from build123d import *

# Parameters (mm, degrees)
SKETCH2_R               = 6
BOSS_EXTRUDE1_DEPTH     = 4
SKETCH3_W               = 5
SKETCH3_H               = 30
BOSS_EXTRUDE3_DEPTH     = 24
BOSS_EXTRUDE5_DEPTH     = 5
SKETCH7_3_R             = 3.25755
CUT_EXTRUDE3_DEPTH      = 5
FILLET3_R               = 10
CUT_EXTRUDE4_DEPTH      = 25
CUT_EXTRUDE4_DEPTH_BACK = 1
SKETCH8_R               = 7.5
CUT_EXTRUDE5_DEPTH      = 50.515905416
CUT_EXTRUDE5_DEPTH_BACK = 50.515905416
SKETCH9_R               = 2.75
FILLET4_R               = 1
BOSS_EXTRUDE6_DEPTH     = 4
FILLET6_R               = 2
BOSS_EXTRUDE7_DEPTH     = 4


with BuildPart() as part:
    # Sketch2 → Boss-Extrude1 (new body)
    with BuildSketch(Plane(origin=(0, 0, 0), x_dir=(1, 0, 0), z_dir=(0, 1, 0))):
        with BuildLine():
            Line((18.000912404, -14.946929254), (18.000912404, 15.053070746))
            Line((18.000912404, 15.053070746), (0.039090451, 15.053070746))
            ThreePointArc((0.039090451, 15.053070746), (-10.199781301, 11.024824414), (-14.94907539, 1.099832277))
            ThreePointArc((-14.94907539, 1.099832277), (-10.959209921, -10.21234771), (0.039090451, -15.000022662))
            Line((0.039090451, -15.000022662), (10.151696986, -14.946929254))
            Line((10.151696986, -14.946929254), (18.000912404, -14.946929254))
        make_face()
        with Locations(Location((0.000957071, 0.012970337, 0), (0, 0, 270))):
            Circle(SKETCH2_R, mode=Mode.SUBTRACT)
    boss_extrude1 = extrude(amount=BOSS_EXTRUDE1_DEPTH)

    # Sketch3 → Boss-Extrude3 (add)
    with BuildSketch(Plane(origin=(0, 4, 0), x_dir=(1, 0, 0), z_dir=(0, 1, 0))):
        with Locations((15.500912404, 0.053070746)):
            Rectangle(SKETCH3_W, SKETCH3_H)
    extrude(amount=BOSS_EXTRUDE3_DEPTH)

    # Mirror1: Boss-Extrude1 across plane
    add(boss_extrude1.mirror(Plane.ZX.offset(16)))

    # Sketch7 → Boss-Extrude5 (add)
    with BuildSketch(Plane.ZY.offset(-13.000912404)):
        with BuildLine():
            Line((-15.053070746, 0), (-15.053070746, 4))
            Line((-15.053070746, 4), (-15.053070746, 7.075913265))
            ThreePointArc((-15.053070746, 7.075913265), (-18.310620746, 10.333463265), (-15.053070746, 13.591013265))
            Line((-15.053070746, 13.591013265), (-15.053070746, 20.666926531))
            ThreePointArc((-15.053070746, 20.666926531), (-25.386534011, 10.333463265), (-15.053070746, 0))
        make_face()
        with BuildLine():
            ThreePointArc((25.146929254, 21.8), (22.159418422, 29.012489168), (14.946929254, 32))
            Line((14.946929254, 32), (14.946929254, 28))
            Line((14.946929254, 28), (14.946929254, 25.05755))
            ThreePointArc((14.946929254, 25.05755), (17.250364949, 24.103435695), (18.204479254, 21.8))
            ThreePointArc((18.204479254, 21.8), (17.250364949, 19.496564305), (14.946929254, 18.54245))
            Line((14.946929254, 18.54245), (14.946929254, 11.6))
            ThreePointArc((14.946929254, 11.6), (22.159418422, 14.587510832), (25.146929254, 21.8))
        make_face()
        with BuildLine():
            Line((14.946929254, 28), (14.946929254, 32))
            ThreePointArc((14.946929254, 32), (4.746929254, 21.8), (14.946929254, 11.6))
            Line((14.946929254, 11.6), (14.946929254, 18.54245))
            ThreePointArc((14.946929254, 18.54245), (11.689379254, 21.8), (14.946929254, 25.05755))
            Line((14.946929254, 25.05755), (14.946929254, 28))
        make_face()
    extrude(amount=-BOSS_EXTRUDE5_DEPTH)

    # Sketch7<3> → Cut-Extrude3 (cut)
    with BuildSketch(Plane.ZY.offset(-13.000912404)):
        with Locations((14.946929254, 21.8)):
            Circle(SKETCH7_3_R)
        with Locations((-15.053070746, 10.333463265)):
            Circle(SKETCH7_3_R)
    extrude(amount=-CUT_EXTRUDE3_DEPTH, mode=Mode.SUBTRACT)

    # Fillet3
    # the kernel refuses this fillet: 10 mm, written as the material it adds along each edge
    with BuildSketch(Plane(origin=(13.000912404, 20.666926531, -15.053070746), x_dir=(0, -0.25425566101904284, -0.9671370424297528), z_dir=(1, 0, 0))) as fillet3_piece_1:
        with BuildLine():
            CenterArc((7.797239676, 9.671370424), FILLET3_R, 194.729484057, 60.541031886)
            Line((-1.874130748, 7.128813814), (0, 0))
            ThreePointArc((0, 0), (2.627341533, 0.339588165), (5.254683066, 0))
        make_face()
    extrude(amount=5)
    with BuildSketch(Plane(origin=(13.000912404, 11.6, 14.946929254), x_dir=(0, -1, 0), z_dir=(1, 0, 0))) as fillet3_piece_2:
        with BuildLine():
            CenterArc((7.351068344, -10), FILLET3_R, 90, 60.326985198)
            ThreePointArc((-1.337579351, -5.04950495), (-0.340063626, -2.611829759), (0, 0))
            Line((0, 0), (7.351068344, 0))
        make_face()
    extrude(amount=5)

    # Sketch8 → Cut-Extrude4 (cut, two sides: drawn at the far end of the back side and taken through both)
    with BuildSketch(Plane(origin=(0, 4, 0), x_dir=(1, 0, 0), z_dir=(0, 1, 0)).offset(-CUT_EXTRUDE4_DEPTH_BACK)):
        with Locations(Location((0, 0, 0), (0, 0, 90))):
            Circle(SKETCH8_R)
    extrude(amount=CUT_EXTRUDE4_DEPTH + CUT_EXTRUDE4_DEPTH_BACK, mode=Mode.SUBTRACT)

    # Sketch9 → Cut-Extrude5 (cut, two sides: drawn at the far end of the back side and taken through both)
    with BuildSketch(Plane.ZY.offset(-13.000912404).offset(-CUT_EXTRUDE5_DEPTH_BACK)):
        with Locations((9, 10.2)):
            Circle(SKETCH9_R)
        with Locations((-9, 21.8)):
            Circle(SKETCH9_R)
    extrude(amount=CUT_EXTRUDE5_DEPTH + CUT_EXTRUDE5_DEPTH_BACK, mode=Mode.SUBTRACT)

    # Fillet4
    fillet4_edges = [part.edges().sort_by_distance(p)[0] for p in [
        (13.000912404, 4, -0.053070746),
        (13.000912404, 28, -0.053070746),
    ]]
    fillet(fillet4_edges, radius=FILLET4_R)

    # Sketch10 → Boss-Extrude6 (add)
    with BuildSketch(Plane.XZ):
        with BuildLine():
            ThreePointArc((0.039090451, -15.053070746), (-5.733491903, -13.900038334), (-10.620178824, -10.617892431))
            Line((-10.620178824, -10.617892431), (-9.005905934, -15.053070746))
            Line((-9.005905934, -15.053070746), (0.039090451, -15.053070746))
        make_face()
        with BuildLine():
            ThreePointArc((-10.571777141, 10.613334735), (-5.701848976, 13.860114152), (0.039090451, 15.000022662))
            Line((0.039090451, 15.000022662), (-8.957960629, 15.047259158))
            Line((-8.957960629, 15.047259158), (-10.571777141, 10.613334735))
        make_face()
    extrude(amount=-BOSS_EXTRUDE6_DEPTH)

    # Fillet6
    fillet6_edges = [part.edges().sort_by_distance(p)[0] for p in [
        (-9.005905934, 2, -15.053070746),
        (-8.957960629, 2, 15.047259158),
    ]]
    fillet(fillet6_edges, radius=FILLET6_R)

    # Sketch11 → Boss-Extrude7 (add)
    with BuildSketch(Plane(origin=(0, 32, 0), x_dir=(1, 0, 0), z_dir=(0, 1, 0))):
        with BuildLine():
            ThreePointArc((0.039090451, -15.000022662), (-5.701848976, -13.860114152), (-10.571777141, -10.613334735))
            Line((-10.571777141, -10.613334735), (-9.439611791, -13.723933469))
            ThreePointArc((-9.439611791, -13.723933469), (-8.703074785, -14.681202997), (-7.549726254, -15.039865618))
            Line((-7.549726254, -15.039865618), (0.039090451, -15.000022662))
        make_face()
        with BuildLine():
            Line((-9.484876099, 13.737111032), (-10.620178824, 10.617892431))
            ThreePointArc((-10.620178824, 10.617892431), (-5.733491903, 13.900038334), (0.039090451, 15.053070746))
            Line((0.039090451, 15.053070746), (-7.605490857, 15.053070746))
            ThreePointArc((-7.605490857, 15.053070746), (-8.75264373, 14.691374834), (-9.484876099, 13.737111032))
        make_face()
    extrude(amount=-BOSS_EXTRUDE7_DEPTH)


solid = part.part
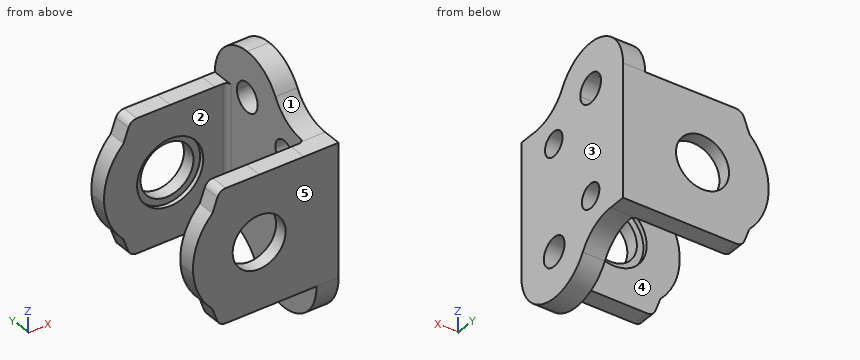
For this review, take the finished solid that the model builds, in its own axes (mm). Face numbers are marked on the shaded views. A direction names the side the tool comes from. Coordinates: 2 decimals unless noted, no trailing zeros. Order: outer loops, then holes, each group sorted by start corner. A loop starts at its lowest first (then second) coordinate and runs counter-clockwise, first axis right, second up. Notation, with made-up numbers: (4.25, 80) - (48.25, 80) arc R30 ccw to (48.25, 113) - close; hole circle Ø5 at (7.25, -17.5). An arc over 180 degrees is marked (long way). Answer as CSV lines item,"result". Start each with the question number.
1) Insertion check: P1, Ø8, axis at x = -3.5, y = 23.5, coming from the +Z side; P2, Ø2.5, axis at x = 2, y = 2, coming from the -Z side; P3, Ø1.4, axis at x = 12, y = 28.5, coming from the +Z side; P4, Ø7, axis at y = 21.8, z = -9, coming from the -X side. Each pin has a flat end and moves straight along its axis. Give the tip position at first contact, or say it passes through.
2) Add section D-D (z = 0). State the section outline as (x, y) points, then the cut area to 3 significant figures.
3) To check wall thickness, follow line 1 along Y through (x, z) = (-8, 3); line 2 along Y through (x, z) = (16.3, 9); line 3 along Z through (x, y) = (16.3, 10.2). State the ranges of each line that lie inside material, in increasing order. Write a range as [from, to].
4) Draft analysis for pull direction Y (two halves, no side actions). For the marked faces 1, 2 and 3, state which applies: +Y half, -Y half, draft (parallel to the pull), parting line (faces both ways), or undercut.
5) Add section A-A (z = -14.5). State the section outline as (x, y) points.
6) Machinability: for the marked faces 4 and 5, which of the approach directions +Z, -Z, +X, -X, +Y, -Y give a long, thin tool a straight path to every point of the face, cutting with its end or side? Answer none if there is none.
7) Add section B-B (x = -11.5). State the section outline as (y, z) points, then the cut area to 3 significant figures.
8) Add section C-C (y = 23). State the section outline as (x, z) points.
Result:
1,P1,"through"
1,P2,"z = -15.05"
1,P3,"z = 14.95"
1,P4,"x = 13"
2,outline,"(-14.99, 0) - (-6, 0) - (-6, 3) - (-7.5, 3) - (-7.5, 4) - (-14.99, 4) - close; (-14.99, 28) - (-7.5, 28) - (-7.5, 29) - (-6, 29) - (-6, 32) - (-14.99, 32) - close; (6, 0) - (18, 0) - (18, 32) - (6, 32) - (6, 29) - (7.5, 29) - (7.5, 28) - (12, 28) arc R1 cw to (13, 27) - (13, 5) arc R1 cw to (12, 4) - (7.5, 4) - (7.5, 3) - (6, 3) - close"
2,area,"282 mm^2"
3,line 1,"[0, 4], [28, 32]"
3,line 2,"[0, 7.45], [12.95, 32]"
3,line 3,"[-25.39, -18.31], [-11.8, 6.25], [11.75, 16.91]"
4,face 1,"-Y half"
4,face 2,"undercut"
4,face 3,"draft"
5,outline,"(-8.99, 0) - (18, 0) - (18, 7.12) - (13, 7.12) - (13, 5) arc R1 cw to (12, 4) - (-8.99, 4) - close; (-8.99, 28) - (12, 28) arc R1 cw to (13, 27) - (13, 13.54) - (18, 13.54) - (18, 32) - (-8.99, 32) - close"
6,face 4,"+Z, -Z, -X"
6,face 5,"+Z, -Z, +X, -X, -Y"
7,outline,"(0, -9.65) - (4, -9.65) - (4, 9.6) - (0, 9.6) - close; (28, -9.65) - (32, -9.65) - (32, 9.6) - (28, 9.6) - close"
7,area,"154 mm^2"
8,outline,"(13, -16.41) - (18, -16.41) - (18, -11.47) - (13, -11.47) - close; (13, -6.53) - (18, -6.53) - (18, 11.92) - (13, 11.92) - close; (13, 17.98) - (18, 17.98) - (18, 25.08) - (13, 25.08) - close"
